Geometry: see drawing. Coordinates: mm, zero at the bounding-box minimum. A direction names the side the tool comes from. Give positions to 0.01 mm unless a question says otherwise; leave off trailing zeros. Order: outer loops, then holes, each group sorted by start corner. A loop starts at its lowest first (then second) coordinate and runs counter-clockwise, first axis right, second up. Notation, with made-up numbers: M 12.25,-27.5 L 53.25,-27.5 A32 cw 53.25,8.5 Z; hole C 12,45.5 d6. An arc over 180 degrees is marked long. Answer as a JSON object with one key per item and string values. Group by question number.
1. Section query B-B (z = 20). Output: boundary loops of the cut face in (x, y), plus the area to 3 significant figures.
2. Section query D-D (x = 5). Output: boundary loops of the cut face in (y, z).
3. Pull-direction query (Z, two-part tool) for the marked faces 3, 4 and 5; classes: +Z half, -Z half, draft (parallel to the pull), parting line (faces both ways), or undercut.
4. Section query C-C (y = 2.75). Output: boundary loops of the cut face in (x, z).
5. Pin query (flat end, axial travel): P1, Ø2, axis at x = 4, y = 6, coming from the -Z side; P2, Ø3, axis at x = 8.5, y = 6, coming from the -Z side; P3, Ø4, axis at y = 5, z = 22, coming from the -X side. Return the tip coordinate at first contact, or that it passes through.
6. Section query A-A (x = 20). Output: boundary loops of the cut face in (y, z), plus the area to 3 significant figures.
7. Material intervals for L1, parallel to Z at x = 20, y = 5.25; L2, parallel to Z at x = 18.5, y = 6.25, sorted ascending. Write a range as [from, to].
8. Set-up query: the marked faces 1 and 2. Return all of +Z, -Z, +X, -X, +Y, -Y with unobstructed straight access to the full face (end or side cutting, diameter ignored); none if empty.
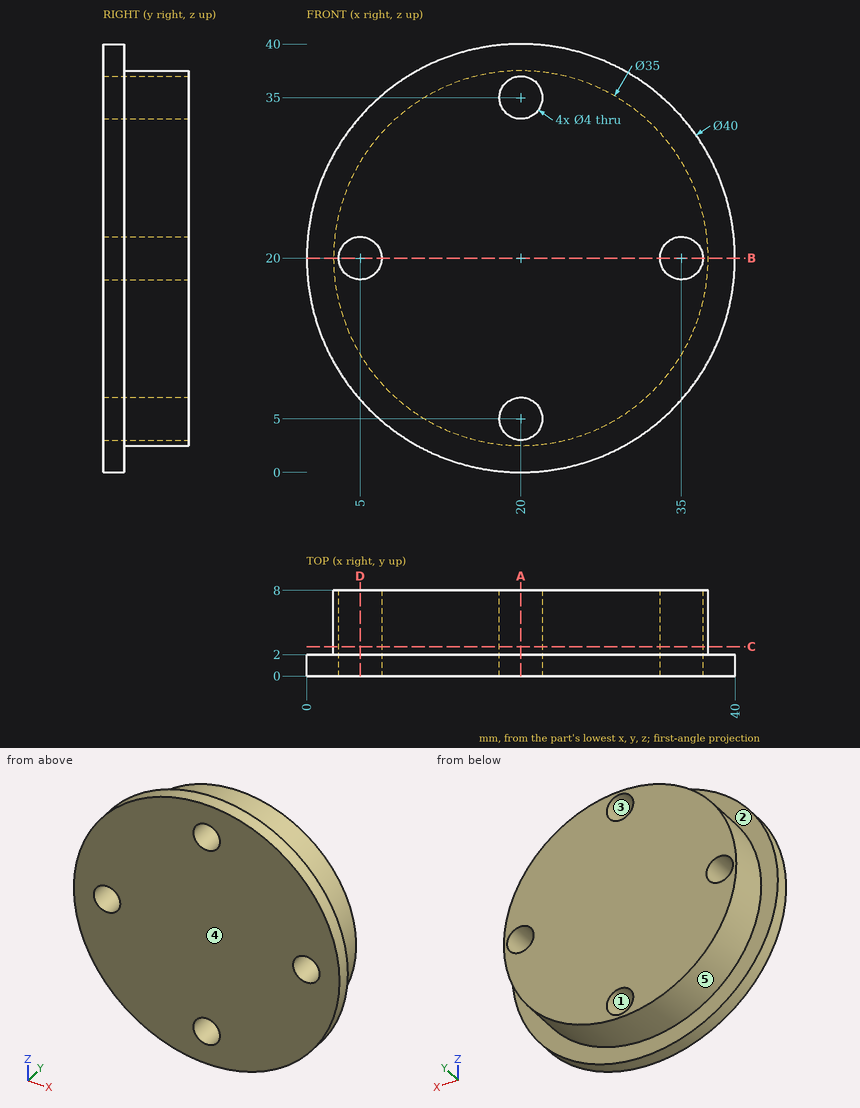
Answer sheet:
{
 "1": {"outline": "M 0,0 L 3,0 L 3,8 L 2.5,8 L 2.5,2 L 0,2 Z; M 7,0 L 33,0 L 33,8 L 7,8 Z; M 37,0 L 40,0 L 40,2 L 37.5,2 L 37.5,8 L 37,8 Z", "area": "226 mm^2"},
 "2": {"outline": "M 0,6.77 L 2,6.77 L 2,10.99 L 8,10.99 L 8,18 L 0,18 Z; M 0,22 L 8,22 L 8,29.01 L 2,29.01 L 2,33.23 L 0,33.23 Z"},
 "3": {"face 3": "undercut", "face 4": "draft", "face 5": "parting line"},
 "4": {"outline": "C 20,20 d35; hole C 5,20 d4; hole C 20,5 d4; hole C 20,35 d4; hole C 35,20 d4"},
 "5": {"P1": "z = 10.99", "P2": "z = 5.64", "P3": "x = 2.5"},
 "6": {"outline": "M 0,0 L 2,0 L 2,2.5 L 8,2.5 L 8,3 L 0,3 Z; M 0,7 L 8,7 L 8,33 L 0,33 Z; M 0,37 L 8,37 L 8,37.5 L 2,37.5 L 2,40 L 0,40 Z", "area": "226 mm^2"},
 "7": {"L1": "[2.5, 3], [7, 33], [37, 37.5]", "L2": "[2.56, 3.68], [6.32, 33.68], [36.32, 37.44]"},
 "8": {"face 1": "+Y, -Y", "face 2": "+Y"}
}
